```python
from build123d import *

# Parameters (mm, degrees)
F1_DEPTH = 15
F2_R     = 7.5
F3_DEPTH = 25
F4_R     = 5
F5_W     = 8.242
F5_H     = 12.533
F6_DEPTH = 10


# Not quite as in the source:
# - a feature names something its author has since deleted; it is built from what else it names


with BuildPart() as f1:
    # F0 (on Top) → F1 (new body)
    with BuildSketch(Plane.XY):
        with BuildLine():
            Line((47.6969600708, 15), (58.0947501931, 15))
            ThreePointArc((58.0947501931, 15), (0, 60), (-58.0947501931, 15))
            Line((-58.0947501931, 15), (-47.6969600708, 15))
            ThreePointArc((-47.6969600708, 15), (0, 50), (47.6969600708, 15))
        make_face()
        with BuildLine():
            Line((-47.6969600708, 15), (-58.0947501931, 15))
            ThreePointArc((-58.0947501931, 15), (-60, 0), (-58.0947501931, -15))
            Line((-58.0947501931, -15), (-47.6969600708, -15))
            ThreePointArc((-47.6969600708, -15), (-50, 0), (-47.6969600708, 15))
        make_face()
        with BuildLine():
            ThreePointArc((-58.0947501931, -15), (0, -60), (58.0947501931, -15))
            Line((58.0947501931, -15), (47.6969600708, -15))
            ThreePointArc((47.6969600708, -15), (0, -50), (-47.6969600708, -15))
            Line((-47.6969600708, -15), (-58.0947501931, -15))
        make_face()
        with BuildLine():
            ThreePointArc((58.0947501931, -15), (59.521781776, -7.560257549), (60, 0))
            ThreePointArc((60, 0), (59.521781776, 7.560257549), (58.0947501931, 15))
            Line((58.0947501931, 15), (47.6969600708, 15))
            ThreePointArc((47.6969600708, 15), (49.4208862908, 7.5878849641), (50, 0))
            ThreePointArc((50, 0), (49.4208862908, -7.5878849641), (47.6969600708, -15))
            Line((47.6969600708, -15), (58.0947501931, -15))
        make_face()
        with BuildLine():
            ThreePointArc((50, 0), (49.4208862908, 7.5878849641), (47.6969600708, 15))
            Line((47.6969600708, 15), (-47.6969600708, 15))
            ThreePointArc((-47.6969600708, 15), (-50, 0), (-47.6969600708, -15))
            Line((-47.6969600708, -15), (47.6969600708, -15))
            ThreePointArc((47.6969600708, -15), (49.4208862908, -7.5878849641), (50, 0))
        make_face()
    extrude(amount=F1_DEPTH)

    # F2 (on face) → F3 (join)
    with BuildSketch(Plane.XY.offset(15)):
        with Locations((-50, 0)):
            Circle(F2_R)
    extrude(amount=F3_DEPTH)

    # F4
    f4_edges = [f1.edges().sort_by_distance(p)[0] for p in [
        (-57.5, 0, 40),
    ]]
    fillet(f4_edges, radius=F4_R)

    # F5 (on face) → F6 (cut)
    with BuildSketch(Plane(origin=(0, 0, 0), x_dir=(1, 0, 0), z_dir=(0, 0, -1))):
        Rectangle(F5_W, F5_H)
    extrude(amount=-F6_DEPTH, mode=Mode.SUBTRACT)


solid = f1.part
```
Check sheet for the modelled part. Datum: model origin and axes. Units: mm. A direction names the side the tool comes from. Give positions to 0.01 mm unless a question says otherwise; leave off trailing zeros. Write each loop counter-clockwise with the first axis right and the second up, starting at its lowest first coordinate (ties: lowest second). Pieces come first, ordered by that corner, then holes. Notation, with made-up numbers: (81, -28.5) -> (114, -28.5) arc R19 cw to (114, -0.5) -> close; hole circle Ø3 at (-12, -36). An arc over 180 degrees is marked (long way). Use CSV: the item, a comma, the result in double quotes. Start each with the question number.
Q1. Cross-section at A-A on y = 20.5. Enter the section's corners in (x, z), and give its area (3 significant figures).
Q2. Cross-section at C-C on x = -7.5. Enter the section's corners in (y, z), and give its area (3 significant figures).
Q3. Cross-section at B-B on z = 7. Enter the section's corners in (x, y).
Q4. Scan lines: line 1 along Y through (x, z) = (-44, 3.5); line 2 along Y through (x, z) = (21.5, 8); line 3 along Z through (x, y) = (-17.5, 52.5). Record each from-to range of solid material in increasing order.
Q5. Release check for a two-part mould opening along Y. For faces 1 (the flat face through (-50, 0, 40)), 2 (the cylindrical face through (-42.846, 2.253, 24.86)), 3 (the flat face through (0, 0, 10)) record: +Y half, -Y half, draft (parallel to the pull), parting line (faces both ways), or undercut.
Q6. Depth check by flat-ended pin: P1, Ø5, axis at y = 0.5, z = 5, coming from the -X side; P2, Ø5, axis at x = -0.5, y = 8, coming from the +Z side; P3, Ø1.5, axis at x = -44, z = 8, coming from the +Y side. Enter the tip coordinate at first touch or a pass-through.
Q7. Tool access check on faces 4 (the flat face through (4.121, 0, 5)), 5 (the flat face through (-1, -12, 0)), 6 (the flat face through (1, 15, 7)). Record the directions out of +Z, -Z, +X, -X, +Y, -Y that give a thin tool (end or side, any length) a straight path to the whole face; none if there is none.
Working result:
1,outline,"(-56.39, 0) -> (-45.6, 0) -> (-45.6, 15) -> (-56.39, 15) -> close; (45.6, 0) -> (56.39, 0) -> (56.39, 15) -> (45.6, 15) -> close"
1,area,"324 mm^2"
2,outline,"(-59.53, 0) -> (-49.43, 0) -> (-49.43, 15) -> (-59.53, 15) -> close; (-15, 0) -> (15, 0) -> (15, 15) -> (-15, 15) -> close; (49.43, 0) -> (59.53, 0) -> (59.53, 15) -> (49.43, 15) -> close"
2,area,"753 mm^2"
3,outline,"circle Ø120 at (0, 0); hole (-47.7, -15) arc R50 ccw to (47.7, -15) -> close; hole (-47.7, 15) -> (47.7, 15) arc R50 ccw to start; hole (-4.12, -6.27) -> (4.12, -6.27) -> (4.12, 6.27) -> (-4.12, 6.27) -> close"
4,line 1,"y = -40.79 to -23.75, -15 to 15, 23.75 to 40.79"
4,line 2,"y = -56.02 to -45.14, -15 to 15, 45.14 to 56.02"
4,line 3,"z = 0 to 15"
5,face 1,"draft"
5,face 2,"parting line"
5,face 3,"undercut"
6,P1,"stops at x = -60"
6,P2,"stops at z = 15"
6,P3,"stops at y = 41.59"
7,face 4,"-Z"
7,face 5,"-Z, +X, -X, +Y, -Y"
7,face 6,"+Z, -Z"
